Geometry: final body of the model. Coordinates: model frame, mm. A direction names the side the tool comes from. Give positions to 0.01 mm unless a question says otherwise; leave off trailing zeros. Order: outer loops, then holes, each group sorted by start corner. A loop starts at its lowest first (then second) coordinate and runs counter-clockwise, first axis right, second up. Notation, with made-up numbers: (30.25, 81.25) - (43.25, 81.25) arc R9 cw to (43.25, 86.25) - close; hole circle Ø9 at (45, 56.5). An arc over 180 degrees is marked (long way). One line per item, written item: value.
```python
from build123d import *

# Parameters (mm, degrees)
BOSS_EXTRUDE1_DEPTH      = 35
BOSS_EXTRUDE1_DEPTH_BACK = 35
CHAMFER1_SIZE            = 10
SKETCH2_R                = 3
CUT_EXTRUDE1_DEPTH       = 35
FILLET1_R                = 3
FILLET2_R                = 4.5
FILLET3_R                = 1


with BuildPart() as part:
    # Sketch1 → Boss-Extrude1 (new body, two sides)
    with BuildSketch(Plane(origin=(0, 0, 0), x_dir=(0, 0, -1), z_dir=(1, 0, 0))) as boss_extrude1_sk:
        Polygon((-21.75, 10), (-21.75, -20), (21.75, -20), (21.75, 40), (16.75, 40), (16.75, -15), (-16.75, -15), (-16.75, 10), align=None)
    extrude(amount=BOSS_EXTRUDE1_DEPTH)
    extrude(boss_extrude1_sk.sketch, amount=-BOSS_EXTRUDE1_DEPTH_BACK)

    # Chamfer1
    chamfer1_edges = [part.edges().sort_by_distance(p)[0] for p in [
        (-35, 40, -19.25),
        (35, 10, 19.25),
        (35, 40, -19.25),
        (-35, 10, 19.25),
    ]]
    chamfer(chamfer1_edges, length=CHAMFER1_SIZE)

    # Sketch2 → Cut-Extrude1 (cut)
    with BuildSketch(Plane.XY.offset(-16.75)):
        with Locations((-20, 24)):
            Circle(SKETCH2_R)
        with Locations((20, 24)):
            Circle(SKETCH2_R)
    extrude(amount=-CUT_EXTRUDE1_DEPTH, mode=Mode.SUBTRACT)

    # Fillet1
    fillet1_edges = [part.edges().sort_by_distance(p)[0] for p in [
        (0, -15, -16.75),
    ]]
    fillet(fillet1_edges, radius=FILLET1_R)

    # Fillet2
    fillet2_edges = [part.edges().sort_by_distance(p)[0] for p in [
        (0, -20, -21.75),
        (0, -20, 21.75),
    ]]
    fillet(fillet2_edges, radius=FILLET2_R)

    # Fillet3
    fillet3_edges = [part.edges().sort_by_distance(p)[0] for p in [
        (0, -15, 16.75),
    ]]
    fillet(fillet3_edges, radius=FILLET3_R)


solid = part.part
```
1) Material intervals for line 1 along Z through (x, y) = (1.5, -7.5); line 2 along Y through (x, z) = (-30, -13); line 3 along Y through (x, z) = (-20, -19), sorted ascending.
Answers below:
line 1: -21.75 to -16.75, 16.75 to 21.75
line 2: -20 to -15
line 3: -19.65 to 21, 27 to 40
2) Section D-D, the plane z = 3.5. Return loops of the section in (x, y).
Answers below:
outline: (-35, -20) - (35, -20) - (35, -15) - (-35, -15) - close
3) Section A-A, the plane x = 20. Return loops of the section in (y, z).
Answers below:
outline: (-20, -17.25) arc R4.5 ccw to (-15.5, -21.75) - (21, -21.75) - (21, -16.75) - (-12, -16.75) arc R3 cw to (-15, -13.75) - (-15, 15.75) arc R1 cw to (-14, 16.75) - (10, 16.75) - (10, 21.75) - (-15.5, 21.75) arc R4.5 ccw to (-20, 17.25) - close; (27, -21.75) - (40, -21.75) - (40, -16.75) - (27, -16.75) - close
4) Section C-C, the plane y = 24. Return loops of the section in (x, z).
Answers below:
outline: (-35, -21.75) - (-23, -21.75) - (-23, -16.75) - (-35, -16.75) - close; (-17, -21.75) - (17, -21.75) - (17, -16.75) - (-17, -16.75) - close; (23, -21.75) - (35, -21.75) - (35, -16.75) - (23, -16.75) - close
5) Mould query, pull axis Z, two halves, no side actions, for faces 1 (the face through (30, 35, -19)), 2 (the face through (0.49, -18.647, -20.467)), 3 (the face through (0.49, -14.14, -15.85)), 4 (the face through (0, -15, 1)). Classes: released by +Z, released by -Z, zero draft, split by the parting line, or undercut.
Answers below:
face 1: zero draft
face 2: released by -Z
face 3: undercut
face 4: undercut
6) Set-up query: faces 5 (the face through (0, 14, -16.75)), 6 (the face through (-30, 5, 19)), 7 (the face through (30, 5, 19)). Return all of +Z, -Z, +X, -X, +Y, -Y with unobstructed straight access to the full face (end or side cutting, diameter ignored); none if empty.
Answers below:
face 5: +X, -X, +Y
face 6: +Z, -X, +Y
face 7: +Z, +X, +Y
7) First-contact query: pin 1 (10 mm diameter, centred on x = 19, y = 21, fed in from +Z); pin 2 (1.5 mm diameter, centred on x = -0.5, z = 20.5, fed in from +Y); pin 3 (15 mm diameter, centred on x = -15, z = 2, fed in from +Y); pin 4 (5 mm diameter, centred on x = -20, y = 24, fed in from -Z). Flat tips, straight axial feed; report the tip coordinate or a pass-through.
Answers below:
pin 1: z = -16.75
pin 2: y = 10
pin 3: y = -15
pin 4: through
8) Section B-B, the plane y = -2. Return loops of the section in (x, z).
Answers below:
outline: (-35, -21.75) - (35, -21.75) - (35, -16.75) - (-35, -16.75) - close; (-35, 16.75) - (35, 16.75) - (35, 21.75) - (-35, 21.75) - close
